Can you work these out from the model? Positions are in its coordinate system, mm. Face numbers are marked on the shaded views. A direction names the side the tool comes from. Give positions to 0.01 mm unless a question says otherwise; leave off trailing zeros. Order: outer loops, then holes, each group sorted by start corner. A loop starts at its lowest first (then second) coordinate and runs counter-clockwise, first axis right, second up. Notation, with made-up numbers: (-16, 53.25) - (-5, 53.25) arc R14 ccw to (-5, 79.25) - close; hole circle Ø11 at (-3.5, 11). An arc over 180 degrees is marked (long way). Return JSON: item names as keys, results as strings.
```python
from build123d import *

# Parameters (mm, degrees)
SKETCH1_R               = 3.175
BOSS_EXTRUDE1_DEPTH     = 20
CUT_EXTRUDE1_DEPTH      = 25
CUT_EXTRUDE1_DEPTH_BACK = 25
SKETCH2_W               = 6.03125
SKETCH2_H               = 91
FILLET1_R               = 10
FILLET2_R               = 5
SKETCH3_R               = 2.38125
CUT_EXTRUDE2_DEPTH      = 6.4


with BuildPart() as part:
    # Sketch1 → Boss-Extrude1 (new body)
    with BuildSketch(Plane.XY):
        with BuildLine():
            Line((-5.85762861, 86.299302532), (-25, 0))
            Line((-25, 0), (-25, -10))
            Line((-25, -10), (25, -10))
            Line((25, -10), (25, 0))
            Line((25, 0), (5.85762861, 86.299302532))
            ThreePointArc((5.85762861, 86.299302532), (0, 91), (-5.85762861, 86.299302532))
        make_face()
        with Locations((0, 85)):
            Circle(SKETCH1_R, mode=Mode.SUBTRACT)
    extrude(amount=BOSS_EXTRUDE1_DEPTH)

    # Sketch2 → Cut-Extrude1 (cut, two sides: drawn at the far end of the back side and taken through both)
    with BuildSketch(Plane(origin=(0, 0, 0), x_dir=(0, 0, -1), z_dir=(1, 0, 0)).offset(-CUT_EXTRUDE1_DEPTH_BACK)):
        with Locations((-16.984375, 45.5)):
            Rectangle(SKETCH2_W, SKETCH2_H)
        with Locations((-3.015625, 45.5)):
            Rectangle(SKETCH2_W, SKETCH2_H)
    extrude(amount=CUT_EXTRUDE1_DEPTH + CUT_EXTRUDE1_DEPTH_BACK, mode=Mode.SUBTRACT)

    # Fillet1
    # the kernel refuses this fillet: 10 mm, written as the material it adds along each edge
    with BuildSketch(Plane(origin=(-25, 0, 13.96875), x_dir=(0, 1, 0), z_dir=(1, 0, 0))) as fillet1_piece_1_section:
        with BuildLine():
            CenterArc((9.178726678, 10), FILLET1_R, 203.382964427, 66.617035573)
            Line((0, 6.03125), (-0.183574534, 5.951875))
            ThreePointArc((-0.183574534, 5.951875), (-0.2, 3.015625), (-0.2, 0))
            Line((-0.2, 0), (0, -0.2))
            Line((0, -0.2), (9.178726678, -0.2))
            Line((9.178726678, -0.2), (9.178726678, 0))
        make_face()
    fillet1_piece_1 = extrude(amount=50, mode=Mode.PRIVATE)
    fillet1_piece_1 = split(fillet1_piece_1, bisect_by=Plane(origin=(23.363313282, 7.378653319, 15.543546825), z_dir=(-0.9762714349563381, -0.2165504220459817, 0)), keep=Keep.TOP, mode=Mode.PRIVATE)
    fillet1_piece_1 = split(fillet1_piece_1, bisect_by=Plane(origin=(-23.363313282, 7.378653319, 15.543546825), z_dir=(0.9762714349563381, -0.2165504220459817, 0)), keep=Keep.TOP, mode=Mode.PRIVATE)
    add(fillet1_piece_1)
    with BuildSketch(Plane(origin=(25, 0, 6.03125), x_dir=(0, 1, 0), z_dir=(-1, 0, 0))) as fillet1_piece_2_section:
        with BuildLine():
            CenterArc((9.178726678, 10), FILLET1_R, 203.382964427, 66.617035573)
            Line((0, 6.03125), (-0.183574534, 5.951875))
            ThreePointArc((-0.183574534, 5.951875), (-0.2, 3.015625), (-0.2, 0))
            Line((-0.2, 0), (0, -0.2))
            Line((0, -0.2), (9.178726678, -0.2))
            Line((9.178726678, -0.2), (9.178726678, 0))
        make_face()
    fillet1_piece_2 = extrude(amount=50, mode=Mode.PRIVATE)
    fillet1_piece_2 = split(fillet1_piece_2, bisect_by=Plane(origin=(23.363313282, 7.378653319, 4.456453175), z_dir=(-0.9762714349563381, -0.2165504220459817, 0)), keep=Keep.TOP, mode=Mode.PRIVATE)
    fillet1_piece_2 = split(fillet1_piece_2, bisect_by=Plane(origin=(-23.363313282, 7.378653319, 4.456453175), z_dir=(0.9762714349563381, -0.2165504220459817, 0)), keep=Keep.TOP, mode=Mode.PRIVATE)
    add(fillet1_piece_2)

    # Fillet2
    # the kernel refuses this fillet: 5 mm, written as the material it takes off along each edge
    with BuildSketch(Plane(origin=(-25, 0, -1.369690533), x_dir=(0, -1, 0), z_dir=(0, 0, 1)), Plane(origin=(25, 0, 21.369690533), x_dir=(0, -1, 0), z_dir=(0, 0, -1))) as fillet2_piece_1:
        with BuildLine():
            CenterArc((FILLET2_R * 0.109575242659, FILLET2_R), FILLET2_R, 257.493496935, 12.506503065)
            Line((-FILLET2_R * 0.106975179387, FILLET2_R * 0.0237285650437), (0, 0))
            Line((0, 0), (FILLET2_R * 0.109575242659, 0))
        make_face()
    extrude(amount=22.739381066, mode=Mode.SUBTRACT)
    with BuildSketch(Plane(origin=(32.111618418, 0, 0), x_dir=(0, 0.5007842597579724, 0.8655721374782461), z_dir=(-1, 0, 0))) as fillet2_piece_2:
        with BuildLine():
            CenterArc((2.903306061, -4.966168801), FILLET2_R, 96.668935359, 53.279164854)
            Line((-1.424554626, -2.462247502), (0, 0))
            ThreePointArc((0, 0), (1.161322425, -0.067662399), (2.322644849, 0))
        make_face()
    extrude(amount=64.223236835, mode=Mode.SUBTRACT)
    with BuildSketch(Plane(origin=(32.111618418, 0, 20), x_dir=(0, -1, 0), z_dir=(-1, 0, 0))) as fillet2_piece_3:
        with BuildLine():
            CenterArc((2.844647367, -5), FILLET2_R, 90, 53.279164854)
            ThreePointArc((-1.163143981, -2.010416667), (-0.523005304, -1.039092598), (0, 0))
            Line((0, 0), (2.844647367, 0))
        make_face()
    extrude(amount=64.223236835, mode=Mode.SUBTRACT)

    # Sketch3 → Cut-Extrude2 (cut)
    with BuildSketch(Plane.XZ.offset(10)):
        with Locations(Location((-15.5, 14.5, 0), (0, 0, 270))):
            Circle(SKETCH3_R)
        with Locations(Location((-15.5, 5.5, 0), (0, 0, 270))):
            Circle(SKETCH3_R)
        with Locations(Location((15.5, 14.5, 0), (0, 0, 270))):
            Circle(SKETCH3_R)
        with Locations(Location((15.5, 5.5, 0), (0, 0, 270))):
            Circle(SKETCH3_R)
    extrude(amount=-CUT_EXTRUDE2_DEPTH, mode=Mode.SUBTRACT)


solid = part.part
```
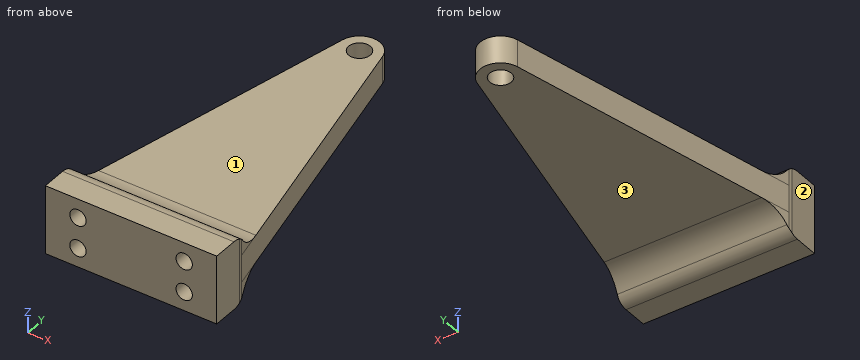
1. Suppose I cut it at A-A (x = 0). List the corners of the cut face in (y, z) for me (3 decimals).
Checks:
{"outline": "(-10, 0) - (-2.845, 0) arc R5 ccw to (1.163, 2.01) arc R10 cw to (9.179, 6.031) - (81.825, 6.031) - (81.825, 13.969) - (9.179, 13.969) arc R10 cw to (1.163, 17.99) arc R5 ccw to (-2.845, 20) - (-10, 20) - close; (88.175, 6.031) - (91, 6.031) - (91, 13.969) - (88.175, 13.969) - close"}
2. Suppose I cut it at D-D (y = 73). List the corners of the cut face in (x, z) for me.
Checks:
{"outline": "(-8.81, 6.03) - (8.81, 6.03) - (8.81, 13.97) - (-8.81, 13.97) - close"}
3. If I drill on L1, parallel to X at y = -4.75, z = 14.5; L2, parallel to Z at x = -15, y = -5; L3, parallel to Y at x = 0, z = 12 (3 decimals), over which ranges is the centre line in solid material (lowest first)? Write a range as [from, to].
Checks:
{"L1": "[-25, -17.88], [-13.12, 13.12], [17.88, 25]", "L2": "[0, 3.17], [7.83, 12.17], [16.83, 20]", "L3": "[-10, 81.825], [88.175, 91]"}
4. Suppose I cut it at C-C (x = -19). List the corners of the cut face in (y, z) for me.
Checks:
{"outline": "(-10, 0) - (-2.84, 0) arc R5 ccw to (1.16, 2.01) arc R10 cw to (9.18, 6.03) - (27.05, 6.03) - (27.05, 13.97) - (9.18, 13.97) arc R10 cw to (1.16, 17.99) arc R5 ccw to (-2.84, 20) - (-10, 20) - close"}
5. On a 3-axis mill with a long thin cutter (end or side, diameter ignored), from which of +Z, -Z, +X, -X, +Y, -Y can I reach the whole of each face in a straight line? I mean the marked faces 1, 2 and 3. Say none if no direction works.
Checks:
{"face 1": "+Z, +X, -X, +Y", "face 2": "+Z, -Z, -X, +Y, -Y", "face 3": "-Z, +X, -X, +Y"}
6. Suppose I cut it at B-B (y = 85). List the corners of the cut face in (x, z) for me (3 decimals), plus the area to 3 significant figures.
Checks:
{"outline": "(-6.146, 6.031) - (-3.175, 6.031) - (-3.175, 13.969) - (-6.146, 13.969) - close; (3.175, 6.031) - (6.146, 6.031) - (6.146, 13.969) - (3.175, 13.969) - close", "area": "47.2 mm^2"}
7. For pin 1 Ø3 at (y, z) = (18.5, 3.5) entering from +X; pin 2 Ø14 at (x, y) = (-7, 65.5) entering from -Z; pin 3 Ø5.5 at (x, z) = (15.5, 14.5) entering from -Y; pin 4 Ø14 at (x, y) = (10.5, 51.5) entering from +Z, each with a flat end and sliding along its axis, tell me the tip position at first contact or that it passes through.
Checks:
{"pin 1": "through", "pin 2": "z = 6.03", "pin 3": "y = -10", "pin 4": "z = 13.97"}
